Design review of the part shown in the three views and the two pictorial views. Dimensions are in mm from the part's minimum x, y and z. A direction names the side the tool comes from. Give positions to 0.01 mm unless a question says otherwise; leave off trailing zeros. Loops run counter-clockwise (first coordinate to the right, second up) from the corner with the lowest first, then second, coordinate; pieces in that order, holes last.
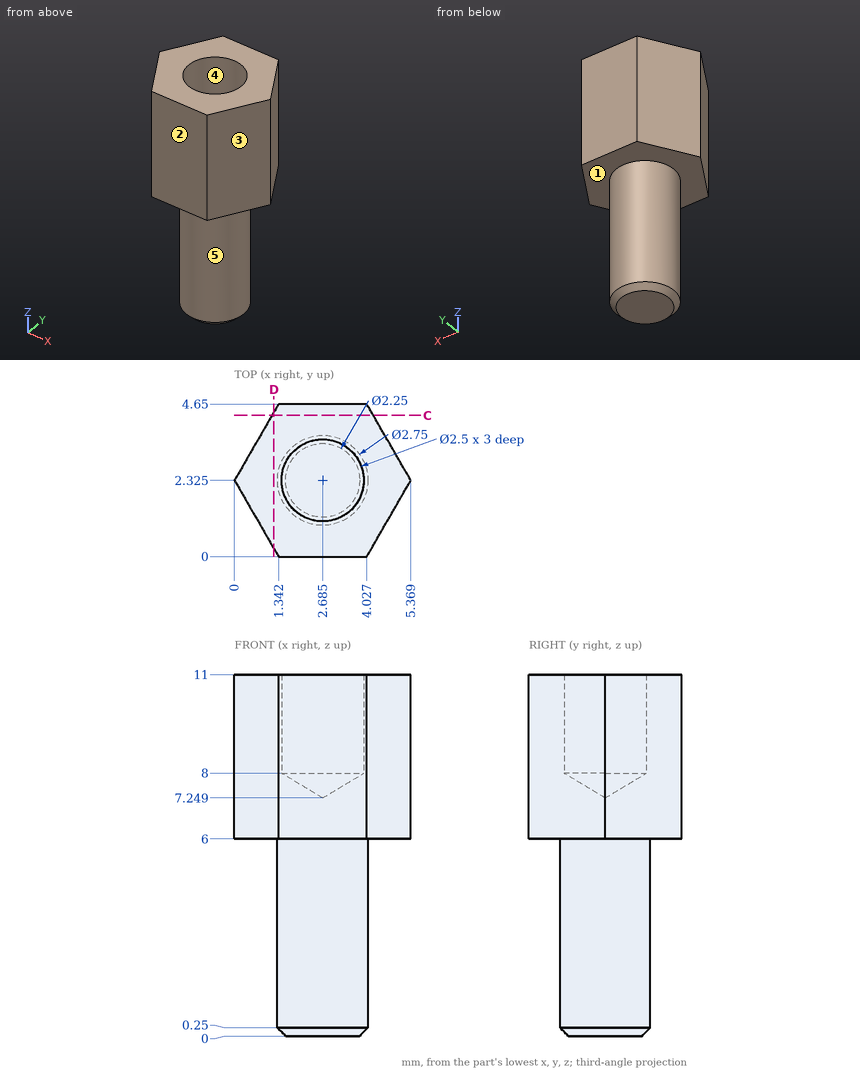
Q1. Tool access review of the marked faces 1 and 2: name each direction out of +Z, -Z, +X, -X, +Y, -Y from which nothing blocks a thin tool from reaching the whole face with its end or side.
Results:
face 1: -Z
face 2: +Z, -Z, +X, -X, -Y
Q2. Take a section at C-C (y = 4.3). Give the boundary of the cut face in (x, z).
Results:
outline: (1.14, 6) - (4.23, 6) - (4.23, 11) - (1.14, 11) - close
Q3. Draft analysis for pull direction X (two halves, no side actions). For the marked faces 3, 4 and 5, state which applies: pulls with the +X half, pulls with the -X half, needs draft (parallel to the pull), parting line crosses it, or undercut.
Results:
face 3: pulls with the +X half
face 4: undercut
face 5: parting line crosses it
Q4. Insertion check: pin 1 (1 mm diameter, centred on x = 4, z = 3, fed in from +Y). The pin has a flat end and moves straight along its axis. Give the tip position at first contact, or say it passes through.
Results:
pin 1: stops at y = 3.43
Q5. Take a section at D-D (x = 1.2). Give the boundary of the cut face in (y, z), plus the area to 3 significant figures.
Results:
outline: (0.25, 6) - (4.4, 6) - (4.4, 11) - (0.25, 11) - close
area: 20.8 mm2
Q6. Wall thickness on line 1 (Z direction, x = 0.55, y = 2.95); line 2 (Y direction, x = 2.9, z = 8.75); line 3 (Y direction, x = 2.7, z = 0.75): over which ranges is each line inside the solid? List them lowest first.
Results:
line 1: z = 6 to 11
line 2: y = 0 to 1.09, 3.56 to 4.65
line 3: y = 0.95 to 3.7
